Design review of the part built by this model. Coordinates are the model's own, in mm. Round coordinates to 2 decimals unless told otherwise and drop trailing zeros. Loops run counter-clockwise (first coordinate to the right, second up) from the corner with the lowest first, then second, coordinate; pieces in that order, holes last. Notation, with made-up numbers: M 76.5,55.25 L 117.5,55.25 A19 cw 117.5,85.25 Z; hole C -31,-33 d2. An arc over 180 degrees is marked long. Use a Markdown table: item, result.
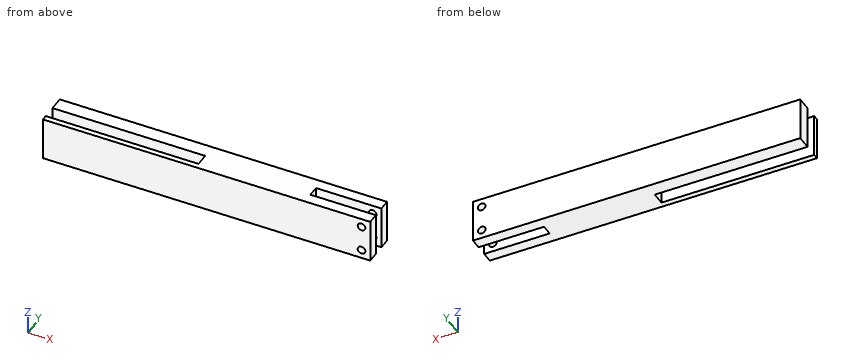
from build123d import *

# Parameters (mm, degrees)
SKETCH1_W           = 150
SKETCH1_H           = 20
BOSS_EXTRUDE3_DEPTH = 15
SKETCH11_W          = 70
SKETCH11_H          = 6
CUT_EXTRUDE5_DEPTH  = 85.961403002
SKETCH12_W          = 30
SKETCH12_H          = 5
CUT_EXTRUDE6_DEPTH  = 85.961403002
SKETCH13_R          = 1.75
CUT_EXTRUDE7_DEPTH  = 84.177160327


with BuildPart() as part:
    # Sketch1 → Boss-Extrude3 (new body)
    with BuildSketch(Plane(origin=(0, 0, 0), x_dir=(1, 0, 0), z_dir=(0, 1, 0))):
        with Locations((-6.2, 0)):
            Rectangle(SKETCH1_W, SKETCH1_H)
    extrude(amount=-BOSS_EXTRUDE3_DEPTH)

    # Sketch11 → Cut-Extrude5 (cut, through all)
    with BuildSketch(Plane.XY.offset(10)):
        with Locations((-46.2, -9.5)):
            Rectangle(SKETCH11_W, SKETCH11_H)
    extrude(amount=-CUT_EXTRUDE5_DEPTH, mode=Mode.SUBTRACT)

    # Sketch12 → Cut-Extrude6 (cut, through all)
    with BuildSketch(Plane.XY.offset(10)):
        with Locations((53.8, -7.5)):
            Rectangle(SKETCH12_W, SKETCH12_H)
    extrude(amount=-CUT_EXTRUDE6_DEPTH, mode=Mode.SUBTRACT)

    # Sketch13 → Cut-Extrude7 (cut, through all)
    with BuildSketch(Plane(origin=(0, 0, 0), x_dir=(1, 0, 0), z_dir=(0, 1, 0))):
        with Locations(Location((64.8, -6, 0), (0, 0, 270))):
            Circle(SKETCH13_R)
        with Locations(Location((64.8, 6, 0), (0, 0, 270))):
            Circle(SKETCH13_R)
    extrude(amount=-CUT_EXTRUDE7_DEPTH, mode=Mode.SUBTRACT)


solid = part.part
1. Take a section at D-D on x = -55.5. Give the boundary of the cut face in (y, z).
Check values:
| item | result |
|---|---|
| outline | M -15,-10 L -12.5,-10 L -12.5,10 L -15,10 Z; M -6.5,-10 L 0,-10 L 0,10 L -6.5,10 Z |
2. Wall thickness on line 1 along Z through (x, y) = (64.8, -12); line 2 along X through (y, z) = (-1.9, -6); line 3 along Y through (x, z) = (-39, -5.5): over which ranges is each line inside the solid? List them lowest first. Write a range as from..to.
Check values:
| item | result |
|---|---|
| line 1 | z = -10..-7.75, -4.25..4.25, 7.75..10 |
| line 2 | x = -81.2..63.05, 66.55..68.8 |
| line 3 | y = -15..-12.5, -6.5..0 |
3. Take a section at C-C on x = 64.8. Give the boundary of the cut face in (y, z).
Check values:
| item | result |
|---|---|
| outline | M -15,-10 L -10,-10 L -10,-7.75 L -15,-7.75 Z; M -15,-4.25 L -10,-4.25 L -10,4.25 L -15,4.25 Z; M -15,7.75 L -10,7.75 L -10,10 L -15,10 Z; M -5,-10 L 0,-10 L 0,-7.75 L -5,-7.75 Z; M -5,-4.25 L 0,-4.25 L 0,4.25 L -5,4.25 Z; M -5,7.75 L 0,7.75 L 0,10 L -5,10 Z |
4. Take a section at A-A on x = 46. Give the boundary of the cut face in (y, z), and give its area (3 significant figures).
Check values:
| item | result |
|---|---|
| outline | M -15,-10 L -10,-10 L -10,10 L -15,10 Z; M -5,-10 L 0,-10 L 0,10 L -5,10 Z |
| area | 200 mm² |
5. Insertion check: pin 1 (1.5 mm diameter, centred on y = -7.5, z = -4, fed in from +X). The pin has a flat end and moves straight along its axis. Give the tip position at first contact, or say it passes through.
Check values:
| item | result |
|---|---|
| pin 1 | stops at x = 38.8 |
6. Take a section at B-B on z = 6. Give the boundary of the cut face in (x, y).
Check values:
| item | result |
|---|---|
| outline | M -81.2,-15 L 63.05,-15 L 63.05,-10 L 38.8,-10 L 38.8,-5 L 63.05,-5 L 63.05,0 L -81.2,0 L -81.2,-6.5 L -11.2,-6.5 L -11.2,-12.5 L -81.2,-12.5 Z; M 66.55,-15 L 68.8,-15 L 68.8,-10 L 66.55,-10 Z; M 66.55,-5 L 68.8,-5 L 68.8,0 L 66.55,0 Z |
